from build123d import *

# Parameters (mm, degrees)
BOSS_EXTRUDE1_DEPTH = 60.2
SKETCH3_R           = 2
CUT_EXTRUDE1_DEPTH  = 20
SKETCH4_W           = 50.2
SKETCH4_H           = 5
CUT_EXTRUDE2_DEPTH  = 20
LPATTERN1_COUNT     = 4
LPATTERN1_PITCH     = 9
FILLET1_R           = 2


with BuildPart() as part:
    # Sketch1 → Boss-Extrude1 (new body)
    with BuildSketch(Plane(origin=(0, 0, 0), x_dir=(0, 0, -1), z_dir=(1, 0, 0))):
        Polygon((0, 0), (0, 15), (44, 15), (44, -20), (42, -20), (42, 13), (10, 13), (10, 3), align=None)
    extrude(amount=-BOSS_EXTRUDE1_DEPTH)

    # Sketch3 → Cut-Extrude1 (cut)
    with BuildSketch(Plane(origin=(0, 0, -44), x_dir=(-1, 0, 0), z_dir=(0, 0, -1))):
        with Locations((54.1, -15)):
            Circle(SKETCH3_R)
        with Locations((54.1, -5)):
            Circle(SKETCH3_R)
        with Locations((6.1, -15)):
            Circle(SKETCH3_R)
        with Locations((6.1, -5)):
            Circle(SKETCH3_R)
        Polygon((9.1, -8), (9.1, 0), (51.1, 0), (51.1, -8), (56.1, -8), (56.1, -12), (51.1, -12), (51.1, -20), (9.1, -20), (9.1, -12), (4.1, -12), (4.1, -8), align=None)
    extrude(amount=-CUT_EXTRUDE1_DEPTH, mode=Mode.SUBTRACT)

    # Sketch4 → Cut-Extrude2 (cut)
    with BuildSketch(Plane(origin=(0, 15, 0), x_dir=(1, 0, 0), z_dir=(0, 1, 0))):
        with Locations((-30.1, 36.5)):
            Rectangle(SKETCH4_W, SKETCH4_H)
    cut_extrude2 = extrude(amount=-CUT_EXTRUDE2_DEPTH, mode=Mode.SUBTRACT)

    # LPattern1: Cut-Extrude2 ×4
    with Locations(*[(0, 0, i * LPATTERN1_PITCH) for i in range(1, LPATTERN1_COUNT)]):
        add(cut_extrude2, mode=Mode.SUBTRACT)

    # Fillet1
    fillet1_edges = [part.edges().sort_by_distance(p)[0] for p in [
        (-30.1, 15, 0),
        (-30.1, 15, -44),
    ]]
    fillet(fillet1_edges, radius=FILLET1_R)


solid = part.part
Source: CAD feature listing. Evaluate the final solid. Frame: model axes, mm. A direction names the side the tool comes from. Round coordinates to 2 decimals unless told otherwise and drop trailing zeros. Loops run counter-clockwise (first coordinate to the right, second up) from the corner with the lowest first, then second, coordinate; pieces in that order, holes last. Notation, with made-up numbers: (18.25, 8) -> (64.25, 8) arc R33 cw to (64.25, 44) -> close; hole circle Ø6 at (64, 68.25). An arc over 180 degrees is marked (long way). Answer as a JSON object with one key per item and string values. Group by question number.
Q1. Mould query, pull axis X, two halves, no side actions, for faces 5 (the flat face through (-30, 9, -7)), 6 (the flat face through (-60.2, 14, -19)), 7 (the flat face through (-30, 4, -42)). Classes: pulls with the +X half, pulls with the -X half, needs draft (parallel to the pull), parting line crosses it, or undercut.
Q2. Ray query, line 1 (Y direction, x = -6, z = -43); line 2 (Y direction, x = -54.1, z = -43.45); line 3 (Z direction, x = -14, y = 8.5). Return the intervals inside material, ascending. Write a range as from..to.
Q3. Access query for faces 1 (the flat face through (-9.1, -16, -43)), 2 (the flat face through (-2, 8, -10)), 3 (the flat face through (-55.2, 14, -18)), 4 (the flat face through (-56.1, -10, -43)). Directions: +Z, -Z, +X, -X, +Y, -Y. A direction counts if a zero-diameter tool reaches every point of the face in a straight line with its end or side. Return the directions, or none.
Q4. Section query A-A (x = -29). Output: boundary loops of the cut face in (y, z).
Q5. Section query B-B (y = -9.5). Output: boundary loops of the cut face in (x, z), plus the area to 3 significant figures.
Q6. Section query C-C (z = -28). Output: boundary loops of the cut face in (x, y), plus the area to 3 significant figures.
Q7. Contact query for flat-ended pins moving along their axis: P1, Ø0.6, axis at x = -32, y = 14, coming from the +Z side; P2, Ø0.6, axis at x = -29, y = 14, coming from the -Z side; P3, Ø10, axis at x = -42.5, z = -37.5, coming from the -Y side. Output: stop coordinate, or through.
Q8. Section query D-D (y = -15). Output: boundary loops of the cut face in (x, z), plus the area to 3 significant figures.
Completed:
{
 "1": {"face 5": "undercut", "face 6": "pulls with the -X half", "face 7": "needs draft"},
 "2": {"line 1": "-20..-17, -13..-12, -8..-7, -3..14.73", "line 2": "-20..-17, -13..-12, -8..-7, -3..14.38", "line 3": "-44..-42, -7..0"},
 "3": {"face 1": "+Z, -Z, -Y", "face 2": "+X, -X, -Y", "face 3": "+Y, -Y", "face 4": "+Z, -Z"},
 "4": {"outline": "(0, -44) -> (13, -44) arc R2 ccw to (15, -42) -> (15, -39) -> (13, -39) -> (13, -42) -> (0, -42) -> close; (0, 0) -> (2.1, -7) -> (15, -7) -> (15, -2) arc R2 ccw to (13, 0) -> close; (13, -34) -> (15, -34) -> (15, -30) -> (13, -30) -> close; (13, -25) -> (15, -25) -> (15, -21) -> (13, -21) -> close; (13, -16) -> (15, -16) -> (15, -12) -> (13, -12) -> close"},
 "5": {"outline": "(-60.2, -44) -> (-56.1, -44) -> (-56.1, -42) -> (-60.2, -42) -> close; (-4.1, -44) -> (0, -44) -> (0, -42) -> (-4.1, -42) -> close", "area": "16.4 mm²"},
 "6": {"outline": "(-60.2, 13) -> (-55.2, 13) -> (-55.2, 15) -> (-60.2, 15) -> close; (-5, 13) -> (0, 13) -> (0, 15) -> (-5, 15) -> close", "area": "20.0 mm²"},
 "7": {"P1": "z = -0.13", "P2": "z = -43.87", "P3": "y = 0"},
 "8": {"outline": "(-60.2, -44) -> (-56.1, -44) -> (-56.1, -42) -> (-60.2, -42) -> close; (-52.1, -44) -> (-51.1, -44) -> (-51.1, -42) -> (-52.1, -42) -> close; (-9.1, -44) -> (-8.1, -44) -> (-8.1, -42) -> (-9.1, -42) -> close; (-4.1, -44) -> (0, -44) -> (0, -42) -> (-4.1, -42) -> close", "area": "20.4 mm²"}
}
